Input: part model. Units: mm. Frame: model coordinates. Face numbers are marked on the shaded views. A direction names the side the tool comes from. Round coordinates to 2 decimals unless told otherwise and drop trailing zeros. Write each loop counter-clockwise with the first axis right and the second up, starting at its lowest first coordinate (ties: lowest second). Pieces come first, ordered by that corner, then holes. Notation, with made-up numbers: M -34,-38 L 2,-38 A21 cw 2,-14 Z; hole C 11.5,-12 d11. An arc over 180 degrees is marked long. Write each question's results on one line, items separated by ' | '. Start each with the question number.
```python
from build123d import *

# Parameters (mm, degrees)
F0_R        = 12.7
F0_R_2      = 9.525
F1_DEPTH    = 25.4
F2_W        = 34.925
F2_H        = 17.78
F2_W_2      = 25.4
F2_H_2      = 12.7
F3_DEPTH    = 2.54
F4_DEPTH    = 20.32
F5_T4_ANGLE = 306.6504874214
F5_T9_ANGLE = 276.2084965167
F6_W        = 12.7
F6_H        = 2.54
F7_DEPTH    = 17.78
F8_R        = 1.190625
F9_DEPTH    = 38.1
F10_W       = 25.4
F10_H       = 5.08
F11_DEPTH   = 12.7


# Not quite as in the source:
# - a fillet or chamfer that OpenCascade refuses, or shapes differently, is made with other operations: its cross-section is extruded or revolved along the edge and cut away or added


with BuildPart() as f1:
    # F0 (on Right) → F1 (new body)
    with BuildSketch(Plane.YZ):
        Circle(F0_R)
        Circle(F0_R_2, mode=Mode.SUBTRACT)
    extrude(amount=-F1_DEPTH)

    # F2 (on Right) → F3 (join)
    with BuildSketch(Plane.YZ):
        with Locations((0, -13.97)):
            Rectangle(F2_W, F2_H)
        with Locations((0, -13.97)):
            Rectangle(F2_W_2, F2_H_2, mode=Mode.SUBTRACT)
        with Locations((0, -13.97)):
            Rectangle(F2_W_2, F2_H_2)
    extrude(amount=F3_DEPTH)

    # F2 (on Right) → F4 (join)
    with BuildSketch(Plane.YZ):
        with Locations((0, -13.97)):
            Rectangle(F2_W, F2_H)
        with Locations((0, -13.97)):
            Rectangle(F2_W_2, F2_H_2, mode=Mode.SUBTRACT)
    extrude(amount=F4_DEPTH)

    # F5: fillet of radius 6.35 on 2 edges, made by hand


with BuildPart() as f5_tool2:
    # F5_s3 → F5_t4 (revolve)
    with BuildSketch(Plane(origin=(0, 0, 0), x_dir=(1, 0, 0), z_dir=(0, 0.8935692652, 0.4489253482))):
        with BuildLine():
            ThreePointArc((-6.35, -9.525), (-1.8598719395, -7.6651280605), (0, -3.175))
            Line((0, -3.175), (0, -9.525))
            Line((0, -9.525), (-6.35, -9.525))
        make_face()
    revolve(axis=Axis((0, 0, 0), (1, 0, 0)), revolution_arc=F5_T4_ANGLE)

    split(bisect_by=Plane.XY.offset(-5.08), keep=Keep.BOTTOM)


with BuildPart() as f1_1:
    add(f1.part)

    # F5_t1: union F5_tool2
    add(f5_tool2.part)


with BuildPart() as f5_tool7:
    # F5_s8 → F5_t9 (revolve)
    with BuildSketch(Plane(origin=(0, 0, 0), x_dir=(1, 0, 0), z_dir=(0, -0.7443610614, 0.6677773658))):
        with BuildLine():
            ThreePointArc((-6.35, 12.7), (-1.8598719395, 14.5598719395), (0, 19.05))
            Line((0, 19.05), (0, 12.7))
            Line((0, 12.7), (-6.35, 12.7))
        make_face()
    revolve(axis=Axis((0, 0, 0), (-1, 0, 0)), revolution_arc=F5_T9_ANGLE)

    split(bisect_by=Plane.XY.offset(-5.08), keep=Keep.BOTTOM)

    split(bisect_by=Plane.XZ.offset(17.4625), keep=Keep.BOTTOM)

    split(bisect_by=Plane.XZ.offset(-17.4625), keep=Keep.TOP)


with BuildPart() as f1_2:
    add(f1_1.part)

    # F5_t6: union F5_tool7
    add(f5_tool7.part)

    # F6 (on face) → F7 (join)
    with BuildSketch(Plane.YZ.offset(20.32)):
        with Locations((0, -6.35)):
            Rectangle(F6_W, F6_H)
    extrude(amount=F7_DEPTH)

    # F8 (on face) → F9 (join)
    with BuildSketch(Plane.YZ.offset(38.1)):
        with BuildLine():
            ThreePointArc((1.927081138, -1.8954984194), (0, -0.508), (-1.927081138, -1.8954984194))
            ThreePointArc((-1.927081138, -1.8954984194), (-3.6249650655, -4.2010485201), (-6.35, -5.08))
            Line((-6.35, -5.08), (6.35, -5.08))
            ThreePointArc((6.35, -5.08), (3.6249650655, -4.2010485201), (1.927081138, -1.8954984194))
        make_face()
        with Locations((0, -2.54)):
            Circle(F8_R, mode=Mode.SUBTRACT)
    extrude(amount=-F9_DEPTH)

    # F10 (on Front) → F11 (cut, symmetric)
    with BuildSketch(Plane.XZ):
        with Locations((19.05, -2.54)):
            Rectangle(F10_W, F10_H)
    extrude(amount=F11_DEPTH, both=True, mode=Mode.SUBTRACT)


solid = f1_2.part
```
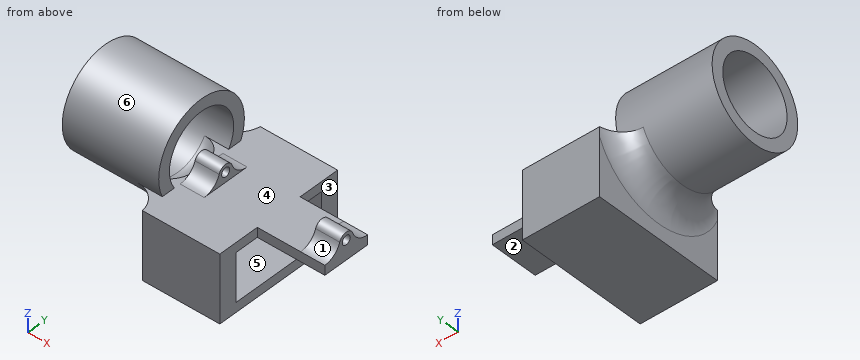
1. Cut plane B-B on z = 7. Output: boundary loops of the cut face in (x, y).
2. Draft query along Y for the marked faces 1, 2 and 3. Return one class per face: +Y half, -Y half, draft (parallel to the pull), parting line (faces both ways), or undercut.
3. Cut plane D-D on x = 29. Output: boundary loops of the cut face in (y, z).
4. Access query for the marked faces 4, 5 and 6. Directions: +Z, -Z, +X, -X, +Y, -Y. A direction counts if a zero-diameter tool reaches every point of the face in a straight line with its end or side. Return the directions, or none.
5. Cut plane C-C on y = 0. Give the number of separate pieces and of enclosed holes in the cut face, and give its area (3 significant figures).
6. Cut plane A-A on x = 7. Output: boundary loops of the cut face in (y, z), and give its area (3 significant figures).
7. Line query: L1, parallel to Z at x = 33, y = 0; L2, parallel to Z at x = 16, y = 7.5; L3, parallel to Y at x = -7, z = 0 (3 decimals). Output: solid intervals per line, ascending. Write a range as from..to.
8. Contact query for flat-ended pins moving along their axis: P1, Ø1.4, axis at y = 2, z = -3.5, coming from the -X side; P2, Ø5.5, axis at x = 13.5, y = -2.5, coming from the +Z side; P3, Ø10, axis at x = 7, z = 4, coming from the +Y side; P4, Ø1.9, axis at y = 0, z = -2.54, coming from the -X side. Output: stop coordinate, or through.
Answers follow:
1) outline: M -25.4,-10.6 L 0,-10.6 L 0,-6.46 L -25.4,-6.46 Z; M -25.4,6.46 L 0,6.46 L 0,10.6 L -25.4,10.6 Z
2) face 1: -Y half | face 2: undercut | face 3: draft
3) outline: M -6.35,-7.62 L 6.35,-7.62 L 6.35,-5.08 L -6.35,-5.08 Z
4) face 4: none | face 5: +X | face 6: -X
5) separate pieces: 4 | enclosed holes: 0 | area: 387 mm2
6) outline: M -17.46,-22.86 L 17.46,-22.86 L 17.46,-5.08 L -17.46,-5.08 Z; hole M -12.7,-20.32 L 12.7,-20.32 L 12.7,-7.62 L -12.7,-7.62 Z | area: 298 mm2
7) L1: z = -7.62..-3.73, -1.35..-0.51 | L2: z = -22.86..-20.32, -7.62..-5.08 | L3: y = -12.7..-9.525, 9.525..12.7
8) P1: stops at x = 0 | P2: stops at z = -5.08 | P3: stops at y = 1.27 | P4: passes through
